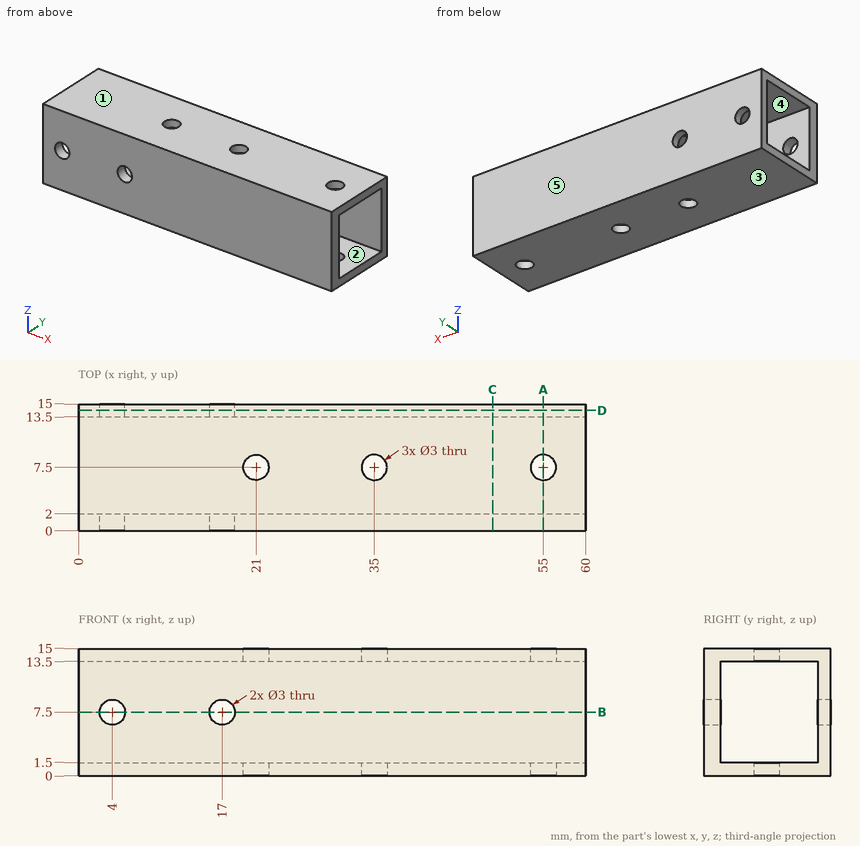
Drawing for the job (mm, zero at the part's lowest x, y, z). A direction names the side the tool comes from. Coordinates: 2 decimals unless noted, no trailing zeros. Order: outer loops, then holes, each group sorted by start corner. A loop starts at its lowest first (then second) coordinate and runs counter-clockwise, first axis right, second up. Notation, with made-up numbers: (16.25, 14) -> (63.25, 14) arc R34 ccw to (63.25, 49) -> close; hole circle Ø8 at (76, 20.25). An arc over 180 degrees is marked (long way). One line per item, written item: value.
(1) Slice it at B-B, the plane z = 7.5. List the corners of the cut face in (x, y), plus the area to 3 significant figures.
Checked values:
outline: (0, 0) -> (2.5, 0) -> (2.5, 2) -> (0, 2) -> close; (0, 13.5) -> (2.5, 13.5) -> (2.5, 15) -> (0, 15) -> close; (5.5, 0) -> (15.5, 0) -> (15.5, 2) -> (5.5, 2) -> close; (5.5, 13.5) -> (15.5, 13.5) -> (15.5, 15) -> (5.5, 15) -> close; (18.5, 0) -> (60, 0) -> (60, 2) -> (18.5, 2) -> close; (18.5, 13.5) -> (60, 13.5) -> (60, 15) -> (18.5, 15) -> close
area: 189 mm2
(2) Drop a flat-ended pin along its axis: pin 1 Ø1.8 at (x, y) = (35, 7.5) entering from -Z. Give the stop position or say it passes through.
Checked values:
pin 1: through
(3) Slice it at A-A, the plane x = 55. List the corners of the cut face in (y, z), plus the area to 3 significant figures.
Checked values:
outline: (0, 0) -> (6, 0) -> (6, 1.5) -> (2, 1.5) -> (2, 13.5) -> (6, 13.5) -> (6, 15) -> (0, 15) -> close; (9, 0) -> (15, 0) -> (15, 15) -> (9, 15) -> (9, 13.5) -> (13.5, 13.5) -> (13.5, 1.5) -> (9, 1.5) -> close
area: 78.0 mm2
(4) Probe line 1 (X direction, y = 14.25, z = 7.5); line 2 (Z direction, x = 31, y = 8.5); line 3 (Y direction, x = 35, z = 14). List the from-to ranges inside material, lowest first. Write a range as [from, to].
Checked values:
line 1: [0, 2.5], [5.5, 15.5], [18.5, 60]
line 2: [0, 1.5], [13.5, 15]
line 3: [0, 6], [9, 15]
(5) Slice it at C-C, the plane x = 49. List the corners of the cut face in (y, z).
Checked values:
outline: (0, 0) -> (15, 0) -> (15, 15) -> (0, 15) -> close; hole (2, 1.5) -> (13.5, 1.5) -> (13.5, 13.5) -> (2, 13.5) -> close
(6) Mould opens along Z. For the marked faces 3, 4 and 5 say: pulls with the +Z half, pulls with the -Z half, needs draft (parallel to the pull), parting line crosses it, or undercut.
Checked values:
face 3: pulls with the -Z half
face 4: undercut
face 5: needs draft
(7) Slice it at D-D, the plane y = 14.25. List the corners of the cut face in (x, z), plus the area to 3 significant figures.
Checked values:
outline: (0, 0) -> (60, 0) -> (60, 15) -> (0, 15) -> close; hole circle Ø3 at (4, 7.5); hole circle Ø3 at (17, 7.5)
area: 886 mm2
(8) Tool access for the marked faces 1 and 2: list every direction of +Z, -Z, +X, -X, +Y, -Y with a clear straight run to the whole face (end or side of a thin tool).
Checked values:
face 1: +Z, +X, -X, +Y, -Y
face 2: +X, -X
